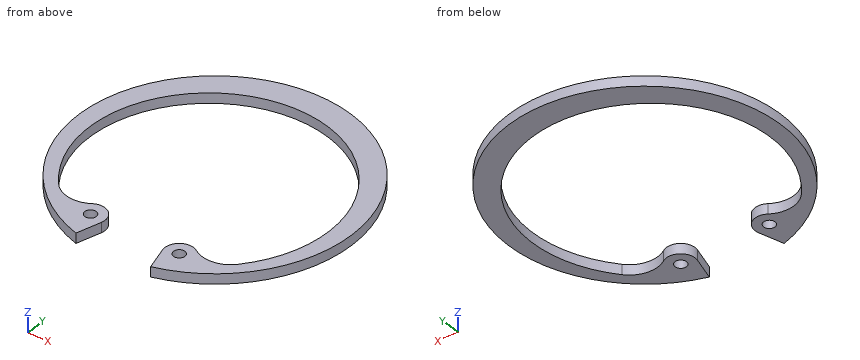
from build123d import *

# Parameters (mm, degrees)
SKETCH2_R           = 1
BOSS_EXTRUDE1_DEPTH = 1.75


with BuildPart() as part:
    # Sketch2 → Boss-Extrude1 (new body)
    with BuildSketch(Plane.XY):
        with BuildLine():
            ThreePointArc((-5.351990622, -18.664609398), (-6.277079647, -15.959251249), (-9.135419395, -15.891087439))
            ThreePointArc((-9.135419395, -15.891087439), (-12.571938491, -16.676326013), (-15.672466243, -14.999128717))
            ThreePointArc((-15.672466243, -14.999128717), (3.5e-08, 19.35), (15.672466197, -14.99912877))
            ThreePointArc((15.672466197, -14.99912877), (12.571938449, -16.676326019), (9.135419383, -15.891087431))
            ThreePointArc((9.135419383, -15.891087431), (6.277079669, -15.959251233), (5.351990603, -18.664609332))
            Line((5.351990603, -18.664609332), (6.546387201, -22.829965279))
            ThreePointArc((6.546387201, -22.829965279), (0, 23.75), (-6.546387201, -22.829965279))
            Line((-6.546387201, -22.829965279), (-5.351990622, -18.664609398))
        make_face()
        with Locations((-7.755144841, -17.975515935)):
            Circle(SKETCH2_R, mode=Mode.SUBTRACT)
        with Locations((7.755144841, -17.975515935)):
            Circle(SKETCH2_R, mode=Mode.SUBTRACT)
    extrude(amount=BOSS_EXTRUDE1_DEPTH)


solid = part.part
Geometry: final body of the model. Coordinates: model frame, mm. Coordinates: 2 decimals unless noted, no trailing zeros. Loops run counter-clockwise (first coordinate to the right, second up) from the corner with the lowest first, then second, coordinate; pieces in that order, holes last. Notation, with made-up numbers: (51, 85) - (108, 85) arc R29 ccw to (108, 106) - close; hole circle Ø2 at (86, 49.5). An arc over 180 degrees is marked (long way). One line per question, with ' | ' between items. Start each with the question number.
(1) Cut plane B-B on x = 17. Output: boundary loops of the cut face in (y, z) (3 decimals), and give its area (3 significant figures).
(2) Ray query, L1, parallel to Y at x = 8, z = 0.1; L2, parallel to X at y = -17.5, z = 0.9; L3, parallel to X at y = -16, z = 0.55. Return the intervals inside material, ascending. Write a range as from..to.
(3) Cut plane A-A on y = -1.4. Output: boundary loops of the cut face in (x, z), and give its area (3 significant figures).
(4) Cut plane D-D on x = 7.5. Output: boundary loops of the cut face in (y, z).
(5) Cut plane C-C on z = 1.45. Output: boundary loops of the cut face in (x, y).
Here are the results:
1) outline: (-16.585, 0) - (-13.298, 0) - (-13.298, 1.75) - (-16.585, 1.75) - close; (10.498, 0) - (16.585, 0) - (16.585, 1.75) - (10.498, 1.75) - close | area: 16.4 mm²
2) L1: -22.36..-18.95, -17.01..-15.49, 17.75..22.36 | L2: -16.06..-8.63, -6.88..-5.3, 5.3..6.88, 8.63..16.06 | L3: -17.55..-14.48, -9.31..-6.22, 6.22..9.31, 14.48..17.55
3) outline: (-23.71, 0) - (-20.75, 0) - (-20.75, 1.75) - (-23.71, 1.75) - close; (20.75, 0) - (23.71, 0) - (23.71, 1.75) - (20.75, 1.75) - close | area: 10.4 mm²
4) outline: (-22.53, 0) - (-18.94, 0) - (-18.94, 1.75) - (-22.53, 1.75) - close; (-17.01, 0) - (-15.49, 0) - (-15.49, 1.75) - (-17.01, 1.75) - close; (17.95, 0) - (22.53, 0) - (22.53, 1.75) - (17.95, 1.75) - close
5) outline: (-15.67, -15) arc R20.75 cw (long way) to (15.67, -15) arc R5 cw to (9.14, -15.89) arc R2.5 ccw to (5.35, -18.66) - (6.55, -22.83) arc R23.75 ccw (long way) to (-6.55, -22.83) - (-5.35, -18.66) arc R2.5 ccw to (-9.14, -15.89) arc R5 cw to start; hole circle Ø2 at (-7.76, -17.98); hole circle Ø2 at (7.76, -17.98)
